from build123d import *

# Parameters (mm, degrees)
ESQUISSE1_R        = 1.5
ESQUISSE1_R_2      = 3
BOSS_EXTRU_1_DEPTH = 5
CONG_3_R           = 1
CONG_7_R           = 1


with BuildPart() as part:
    # Esquisse1 → Boss.-Extru.1 (new body)
    with BuildSketch(Plane.XY):
        with BuildLine():
            Line((10.585988002, 5.428041782), (10.585988002, -2.326303621))
            ThreePointArc((10.585988002, -2.326303621), (7.77052424, -5.304066258), (4.639803855, -2.659733377))
            ThreePointArc((4.639803855, -2.659733377), (-11.05816252, 7.956045933), (-5, -10))
            Line((-5, -10), (5.93338076, -10))
            ThreePointArc((5.93338076, -10), (12.052569379, -7.638961176), (15, -1.779641556))
            Line((15, -1.779641556), (15, 0))
            Line((15, 0), (15, 7.057325334))
            ThreePointArc((15, 7.057325334), (12.225325109, 7.780597138), (10.585988002, 5.428041782))
        make_face()
        with Locations((-5, -7.5)):
            Circle(ESQUISSE1_R, mode=Mode.SUBTRACT)
        with Locations((-5, 0)):
            Circle(ESQUISSE1_R_2, mode=Mode.SUBTRACT)
        with Locations((-5, 7.5)):
            Circle(ESQUISSE1_R, mode=Mode.SUBTRACT)
    extrude(amount=BOSS_EXTRU_1_DEPTH)

    # Congé3
    cong_3_edges = [part.edges().sort_by_distance(p)[0] for p in [
        (15, 7.057325334, 2.5),
    ]]
    fillet(cong_3_edges, radius=CONG_3_R)

    # Congé7
    cong_7_edges = [part.edges().sort_by_distance(p)[0] for p in [
        (4.639803855, -2.659733377, 2.5),
    ]]
    fillet(cong_7_edges, radius=CONG_7_R)


solid = part.part
Verification items for the finished model (mm, model axes). A direction names the side the tool comes from. Coordinates: 2 decimals unless noted, no trailing zeros. Loops run counter-clockwise (first coordinate to the right, second up) from the corner with the lowest first, then second, coordinate; pieces in that order, holes last. Notation, with made-up numbers: (79, 43) -> (105, 43) arc R30 ccw to (105, 67) -> close; hole circle Ø3 at (87, 38.25). An arc over 180 degrees is marked (long way). Answer as a JSON object with one key per item and string values. Group by question number.
Item 1: Sectioned sample at C-C on z = 1.5. State how many separate pieces and enclosed holes the cut face has, plus the area to 3 significant figures.
Item 2: Depth check by flat-ended pin: pin 1 (1 mm diameter, centred on x = -10.5, z = 3, fed in from -Y); pin 2 (3 mm diameter, centred on x = -1.5, z = 3, fed in from +Y); pin 3 (3 mm diameter, centred on y = -3, z = 1, fed in from -X). Enter the tip coordinate at first touch or a pass-through.
Item 3: Sectioned sample at A-A on y = 0. Record the boundary of the cut face in (x, z), plus the area to 3 significant figures.
Item 4: Mould release check, pull along Y, two halves, no side actions. Record for faces 3 (the flat face through (0, 0, 0)), 4 (the cylindrical face through (-2.14, 0.9, 2.46)), 5 (the cylindrical face through (11.983, -7.702, 2.465)): +Y half, -Y half, draft (parallel to the pull), parting line (faces both ways), or undercut.
Item 5: Scan lines: probe 1 along Y at (x, z) = (-5, 3.85); probe 2 along X at (y, z) = (1.5, 4.5); probe 3 along X at (y, z) = (-2.25, 1.4). Record each from-to range of solid material in increasing order.
Item 6: Sectioned sample at D-D on y = 4.5. Record the boundary of the cut face in (x, z), plus the area to 3 significant figures.
Item 7: Tool access check on faces 1 (the flat face through (10.586, 2, 2)), 2 (the flat face through (0, 0, 5)). Record the directions out of +Z, -Z, +X, -X, +Y, -Y that give a thin tool (end or side, any length) a straight path to the whole face; none if there is none.
Item 8: Sectioned sample at B-B on y = -4.5. Record the boundary of the cut face in (x, z), plus the area to 3 significant figures.
Evaluation:
{
 "1": {"separate pieces": "1", "enclosed holes": "3", "area": "382 mm²"},
 "2": {"pin 1": "stops at y = -8.66", "pin 2": "stops at y = 9.8", "pin 3": "stops at x = -14.89"},
 "3": {"outline": "(-15, 0) -> (-8, 0) -> (-8, 5) -> (-15, 5) -> close; (-2, 0) -> (5, 0) -> (5, 5) -> (-2, 5) -> close; (10.59, 0) -> (15, 0) -> (15, 5) -> (10.59, 5) -> close", "area": "92.1 mm²"},
 "4": {"face 3": "draft", "face 4": "undercut", "face 5": "-Y half"},
 "5": {"probe 1": "y = -10 to -9, -6 to -3, 3 to 6, 9 to 10", "probe 2": "x = -14.89 to -7.6, -2.4 to 4.89, 10.59 to 15", "probe 3": "x = -14.74 to -6.98, -3.02 to 4.74, 10.59 to 14.94"},
 "6": {"outline": "(-13.93, 0) -> (3.93, 0) -> (3.93, 5) -> (-13.93, 5) -> close; (10.59, 0) -> (15, 0) -> (15, 5) -> (10.59, 5) -> close", "area": "111 mm²"},
 "7": {"face 1": "+Z, -Z, +Y", "face 2": "+Z, +X, -X, +Y, -Y"},
 "8": {"outline": "(-13.93, 0) -> (5.56, 0) -> (5.56, 5) -> (-13.93, 5) -> close; (9.65, 0) -> (14.3, 0) -> (14.3, 5) -> (9.65, 5) -> close", "area": "121 mm²"}
}
